CAD build for the part. Positions are in the model's coordinates, mm. Face numbers are marked on the shaded views. A direction names the side the tool comes from. Give positions to 0.01 mm unless a question says otherwise; leave off trailing zeros. Order: outer loops, then holes, each group sorted by start corner. A loop starts at its lowest first (then second) coordinate and runs counter-clockwise, first axis right, second up.
Item 1: Band-saw the part on A-A on z = 12.25. Give the cut face in (x, y).
Item 2: Band-saw the part on C-C on x = 13. Give the cut face in (y, z), plus the area to 3 significant figures.
Item 3: Wall check: L1, parallel to X at y = -37.5, z = 5.5; L2, parallel to Y at x = 87, z = 12.25; L3, parallel to Z at x = 53.5, y = -45.5. Give the ranges that are in metal, low to high.
Item 4: Flat gauge pin, fed straight in: P1, Ø17.5, axis at x = 67.5, y = -19, coming from the +Z side. Where does the tip first touch, or does it go through?
Item 5: Which spindle directions (+Z, -Z, +X, -X, +Y, -Y) get a long thin tool onto all of the face, cutting with end or side? Do the marked faces 1 and 2. Say none if no direction does.
Item 6: Band-saw the part on B-B on y = -3. Give the cut face in (x, z).
Item 7: Two-plate mould, pull along X, no slides. Class the marked faces 3, 4 and 5: released by +X, released by -X, zero draft, split by the parting line, or undercut.
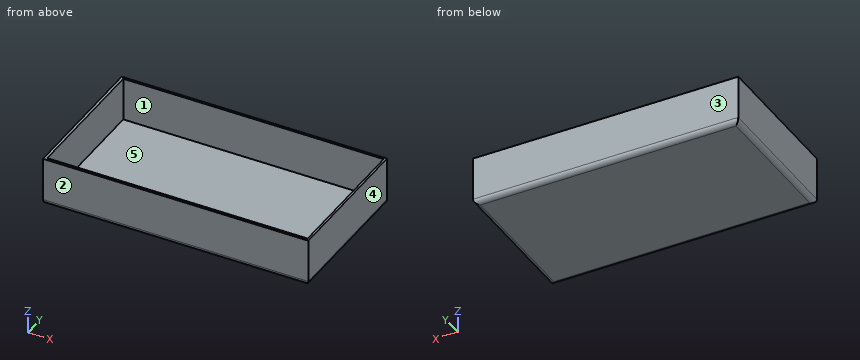
```python
from build123d import *

# Parameters (mm, degrees)
SKETCH_W     = 110
SKETCH_H     = 60
PAD_DEPTH    = 20
SKETCH001_W  = 108
SKETCH001_H  = 58
POCKET_DEPTH = 18
FILLET_R     = 2


with BuildPart() as part:
    # Sketch → Pad (new body)
    with BuildSketch(Plane.XY):
        with Locations((46.444008, -19.812599)):
            Rectangle(SKETCH_W, SKETCH_H)
    extrude(amount=PAD_DEPTH)

    # Sketch001 (on Face6 of Pad) → Pocket (cut)
    with BuildSketch(Plane.XY.offset(20)):
        with Locations((46.57238, -19.707021)):
            Rectangle(SKETCH001_W, SKETCH001_H)
    extrude(amount=-POCKET_DEPTH, mode=Mode.SUBTRACT)

    # Fillet
    fillet_edges = [part.edges().sort_by_distance(p)[0] for p in [
        (46.444008, 10.187401, 0),
        (101.444008, -19.812599, 0),
        (46.444008, -49.812599, 0),
        (-8.555992, -19.812599, 0),
    ]]
    fillet(fillet_edges, radius=FILLET_R)


solid = part.part
```
The answers:
1. outline: (-8.56, -49.81) - (101.44, -49.81) - (101.44, 10.19) - (-8.56, 10.19) - close; hole (-7.43, -48.71) - (100.57, -48.71) - (100.57, 9.29) - (-7.43, 9.29) - close
2. outline: (-49.81, 2) arc R2 ccw to (-47.81, 0) - (8.19, 0) arc R2 ccw to (10.19, 2) - (10.19, 20) - (9.29, 20) - (9.29, 2) - (-48.71, 2) - (-48.71, 20) - (-49.81, 20) - close
2. area: 154 mm2
3. L1: x = -8.56 to -7.43, 100.57 to 101.44
3. L2: y = -49.81 to -48.71, 9.29 to 10.19
3. L3: z = 0 to 2
4. P1: stops at z = 2
5. face 1: +Z
5. face 2: +Z, -Z, +X, -X, -Y
6. outline: (-8.56, 2) arc R2 ccw to (-6.56, 0) - (99.44, 0) arc R2 ccw to (101.44, 2) - (101.44, 20) - (100.57, 20) - (100.57, 2) - (-7.43, 2) - (-7.43, 20) - (-8.56, 20) - close
7. face 3: zero draft
7. face 4: released by +X
7. face 5: undercut
